```python
from build123d import *

# Parameters (mm, degrees)
F1_DEPTH = 152.4
F3_DEPTH = 76.2


with BuildPart() as f1:
    # F0 (on Front) → F1 (new body)
    with BuildSketch(Plane.XZ):
        Polygon((-228.6, 0), (0, 0), (0, 76.2), (-100.878969, 76.2), (-101.6, 152.4), (-228.6, 152.4), align=None)
        Polygon((-100.878969, 76.2), (0, 76.2), (-101.6, 152.4), align=None)
    extrude(amount=F1_DEPTH)

    # F2 (on face) → F3 (cut)
    with BuildSketch(Plane(origin=(0, 0, 0), x_dir=(-1, 0, 0), z_dir=(0, 1, 0))):
        Polygon((101.6, 152.4), (0, 76.2), (101.6, 76.2), align=None)
    extrude(amount=-F3_DEPTH, mode=Mode.SUBTRACT)


solid = f1.part
```
The listing builds one solid part. Answer for the finished solid, in the listing's coordinates (mm). A direction names the side the tool comes from. Give positions to 0.01 mm unless a question says otherwise; leave off trailing zeros. Order: outer loops, then holes, each group sorted by start corner. A loop starts at its lowest first (then second) coordinate and runs counter-clockwise, first axis right, second up.
1) Find section C-C on x = -18. Write down the section's boundary in (y, z).
Reported:
outline: (-152.4, 0) - (0, 0) - (0, 76.2) - (-76.2, 76.2) - (-76.2, 89.7) - (-152.4, 89.7) - close
2) Find section B-B on y = -124.5. Write down the section's boundary in (x, z).
Reported:
outline: (-228.6, 0) - (0, 0) - (0, 76.2) - (-101.6, 152.4) - (-228.6, 152.4) - close
3) For faces 1 (the face through (-164, -75, 152.4)), 2 (the face through (-101.6, -38, 114)), determine the directions among +Z, -Z, +X, -X, +Y, -Y from which every point of the face is accessible in a straight line to the end or side of a thin tool.
Reported:
face 1: +Z, +X, -X, +Y, -Y
face 2: +Z, +X, +Y
4) Given P1, Ø6, axis at y = -123.5, z = 135, coming from the +X side; P2, Ø23, axis at x = -41.5, z = 101.5, coming from the +Y side, each flat-ended and moving along its own axis, determine where each tip first touches the part or whether it passes through.
Reported:
P1: stops at x = -74.4
P2: stops at y = -76.2
5) Find section A-A on x = -84. Write down the section's boundary in (y, z), then the cut area to 3 significant figures.
Reported:
outline: (-152.4, 0) - (0, 0) - (0, 76.2) - (-76.2, 76.2) - (-76.2, 139.2) - (-152.4, 139.2) - close
area: 16,400 mm2
6) Consider line 1 along Z through (x, y) = (-28.5, -47); line 2 along Y through (x, z) = (-77, 115); line 3 along X through (y, z) = (-31, 80). Determine where each line is inside the solid, lowest interval first.
Reported:
line 1: z = 0 to 76.2
line 2: y = -152.4 to -76.2
line 3: x = -228.6 to -101.6
